```python
from build123d import *

# Parameters (mm, degrees)
SKETCH1_W              = 60.96
SKETCH1_H              = 50.8
BOSS_EXTRUDE1_DEPTH    = 40.64
SKETCH3_W              = 60.96
SKETCH3_H              = 50.8
BOSS_EXTRUDE2_DEPTH    = 1.5875
SKETCH2_R              = 18.8
CUT_EXTRUDE1_DEPTH     = 57.785
SKETCH4_W              = 60.96
SKETCH4_H              = 50.8
BOSS_EXTRUDE3_DEPTH    = 3.175
SKETCH6_R              = 9.144
CUT_EXTRUDE2_DEPTH     = 3.175
SKETCH7_R              = 1.5
CUT_EXTRUDE3_DEPTH     = 3.175
SKETCH8_R              = 4.7625
BOSS_EXTRUDE4_DEPTH    = 8.89
CUT_EXTRUDE4_START     = -7.1501
CUT_EXTRUDE4_OUTLINE_R = 4.7625
CUT_EXTRUDE4_DEPTH     = 0.7366
SKETCH9_R              = 4.4704
BOSS_EXTRUDE5_DEPTH    = 0.7366
SKETCH13_R             = 2.54
CUT_EXTRUDE6_DEPTH     = 3.175
SKETCH14_W             = 50.8
SKETCH14_H             = 30.1625
CUT_EXTRUDE7_DEPTH     = 25.4


# Read off the part's stored shape, not the designer's step: Cut-Extrude4
with BuildPart() as part:
    # Sketch1 → Boss-Extrude1 (new body)
    with BuildSketch(Plane(origin=(0, 0, 0), x_dir=(1, 0, 0), z_dir=(0, 1, 0))):
        Rectangle(SKETCH1_W, SKETCH1_H)
    extrude(amount=BOSS_EXTRUDE1_DEPTH)

    # Sketch3 → Boss-Extrude2 (add)
    with BuildSketch(Plane(origin=(0, 0, 0), x_dir=(-1, 0, 0), z_dir=(0, -1, 0))):
        Rectangle(SKETCH3_W, SKETCH3_H)
    extrude(amount=BOSS_EXTRUDE2_DEPTH)

    # Sketch2 → Cut-Extrude1 (cut)
    with BuildSketch(Plane(origin=(30.48, 0, 0), x_dir=(0, 0, -1), z_dir=(1, 0, 0))):
        with Locations((0, 19.812)):
            Circle(SKETCH2_R)
    extrude(amount=-CUT_EXTRUDE1_DEPTH, mode=Mode.SUBTRACT)

    # Sketch4 → Boss-Extrude3 (add)
    with BuildSketch(Plane(origin=(0, 40.64, 0), x_dir=(1, 0, 0), z_dir=(0, 1, 0))):
        Rectangle(SKETCH4_W, SKETCH4_H)
    extrude(amount=BOSS_EXTRUDE3_DEPTH)

    # Sketch6 → Cut-Extrude2 (cut)
    with BuildSketch(Plane.ZY.offset(30.48)):
        with Locations((0, 19.812)):
            Circle(SKETCH6_R)
    extrude(amount=-CUT_EXTRUDE2_DEPTH, mode=Mode.SUBTRACT)

    # Sketch7 → Cut-Extrude3 (cut)
    with BuildSketch(Plane.ZY.offset(30.48)):
        with Locations((0, 32.312000019)):
            Circle(SKETCH7_R)
        with Locations((0, 7.311999981)):
            Circle(SKETCH7_R)
    extrude(amount=-CUT_EXTRUDE3_DEPTH, mode=Mode.SUBTRACT)

    # Sketch8 → Boss-Extrude4 (add)
    with BuildSketch(Plane.XZ.offset(1.5875)):
        with Locations(Location((0, 0, 0), (0, 0, 90))):
            Circle(SKETCH8_R)
    extrude(amount=BOSS_EXTRUDE4_DEPTH)

    # Cut-Extrude4 outline → Cut-Extrude4 (cut)
    with BuildSketch(Plane(origin=(0, 0, 0), x_dir=(1, 0, 0), z_dir=(0, 1, 0)).offset(CUT_EXTRUDE4_START)):
        Circle(CUT_EXTRUDE4_OUTLINE_R)
    extrude(amount=CUT_EXTRUDE4_DEPTH, mode=Mode.SUBTRACT)

    # Sketch9 → Boss-Extrude5 (add)
    with BuildSketch(Plane(origin=(0, -6.4135, 0), x_dir=(-1, 0, 0), z_dir=(0, -1, 0))):
        with Locations(Location((0, 0, 0), (0, 0, 90))):
            Circle(SKETCH9_R)
    extrude(amount=BOSS_EXTRUDE5_DEPTH)

    # Sketch13 → Cut-Extrude6 (cut)
    with BuildSketch(Plane.ZY.offset(30.48)):
        with Locations((8.838834778, 28.650834778)):
            Circle(SKETCH13_R)
        with Locations((-8.838834778, 28.650834778)):
            Circle(SKETCH13_R)
        with Locations((-8.838834778, 10.973165222)):
            Circle(SKETCH13_R)
        with Locations((8.838834778, 10.973165222)):
            Circle(SKETCH13_R)
    extrude(amount=-CUT_EXTRUDE6_DEPTH, mode=Mode.SUBTRACT)

    # Sketch14 → Cut-Extrude7 (cut)
    with BuildSketch(Plane(origin=(30.48, 0, 0), x_dir=(0, 0, -1), z_dir=(1, 0, 0))):
        with Locations((0, 28.73375)):
            Rectangle(SKETCH14_W, SKETCH14_H)
    extrude(amount=-CUT_EXTRUDE7_DEPTH, mode=Mode.SUBTRACT)


solid = part.part
```
Input: part model. Units: mm. Frame: model coordinates. A direction names the side the tool comes from. Coordinates: 2 decimals unless noted, no trailing zeros. Loops run counter-clockwise (first coordinate to the right, second up) from the corner with the lowest first, then second, coordinate; pieces in that order, holes last. Notation, with made-up numbers: M 63,5.5 L 114,5.5 A7 ccw 114,17.5 Z; hole C 71,80 d7. An arc over 180 degrees is marked long. Use a Markdown table: item, result. Add a question column.
1) Section A-A, the plane z = 0. Give the number of separate pieces and of enclosed holes in the cut face, plus the area to 3 significant figures.
2) Set-up query: faces 1 (the flat face through (-27.305, 16, 9)), 2 (the flat face through (5.08, 39, 0)), 3 (the cylindrical face through (-1.431, -8.791, 4.543)), 4 (the cylindrical face through (-28.91, 31.17, 8.51)). Return all of +Z, -Z, +X, -X, +Y, -Y with unobstructed straight access to the full face (end or side cutting, diameter ignored); none if empty.
3) Section B-B, the plane y = 27. Return the cut outline in (x, z) (3 decimals).
4) Pin query (flat end, axial travel): P1, Ø15, axis at y = 34, z = -5.5, coming from the +X side; P2, Ø8.5, axis at x = 22.5, z = 23, coming from the +Y side; P3, Ø12, axis at y = 28.5, z = -9, coming from the -X side; P4, Ø1, axis at x = -3, z = 12.5, coming from the -Y side. Return the tip coordinate at first contact, or that it passes through.
5) Line query: L1, parallel to Y at x = -29, z = 0 (1 decimal); L2, parallel to Y at x = -9, z = 0 (1 decimal); L3, parallel to X at y = 39, z = 0. Output: solid intervals per line, ascending. Write a range as from..to.
6) Draft query along Z for faces 5 (the flat face through (-7, 16, 25.4)), 6 (the cylindrical face through (-1.431, -3.967, 4.543)), 7 (the cylindrical face through (-28.91, 31.17, -9.17)). Return one class per face: +Z half, -Z half, draft (parallel to the pull), parting line (faces both ways), or undercut.
7) Section D-D, the plane y = 16. Return the cut outline in (x, z) (3 decimals), plus the area to 3 significant figures.
Answer below:
| question | item | result |
|---|---|---|
| 1 | separate pieces | 4 |
| 1 | enclosed holes | 0 |
| 1 | area | 470 mm2 |
| 2 | face 1 | +X |
| 2 | face 2 | +Z, -Z, +X, +Y |
| 2 | face 3 | -Y |
| 2 | face 4 | +X, -X |
| 3 | outline | M -30.48,-25.4 L 5.08,-25.4 L 5.08,-17.372 L -27.305,-17.372 L -27.305,-10.769 L -30.48,-10.769 Z; M -30.48,-6.908 L -27.305,-6.908 L -27.305,-5.652 L -30.48,-5.652 Z; M -30.48,5.652 L -27.305,5.652 L -27.305,6.908 L -30.48,6.908 Z; M -30.48,10.769 L -27.305,10.769 L -27.305,17.372 L 5.08,17.372 L 5.08,25.4 L -30.48,25.4 Z |
| 4 | P1 | x = 5.08 |
| 4 | P2 | y = 13.65 |
| 4 | P3 | x = -30.48 |
| 4 | P4 | y = -1.59 |
| 5 | L1 | -1.6..5.8, 8.8..10.7, 29..30.8, 33.8..43.8 |
| 5 | L2 | -1.6..1, 38.6..43.8 |
| 5 | L3 | -30.48..5.08 |
| 6 | face 5 | +Z half |
| 6 | face 6 | parting line |
| 6 | face 7 | undercut |
| 7 | outline | M -30.48,-25.4 L 5.08,-25.4 L 5.08,-18.409 L -27.305,-18.409 L -27.305,-8.312 L -30.48,-8.312 Z; M -30.48,8.312 L -27.305,8.312 L -27.305,18.409 L 5.08,18.409 L 5.08,25.4 L -30.48,25.4 Z |
| 7 | area | 561 mm2 |
